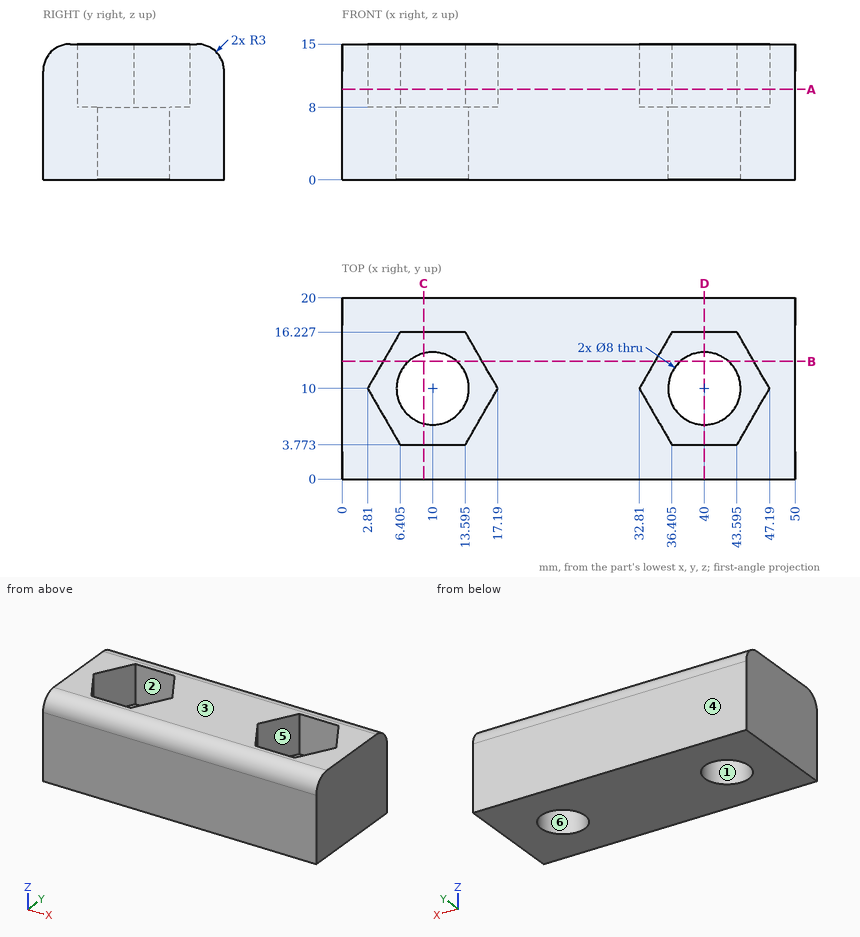
Can you work these out from the drawing? Everything is in mm from the part's minimum corner. A direction names the side the tool comes from. Coordinates: 2 decimals unless noted, no trailing zeros. Loops run counter-clockwise (first coordinate to the right, second up) from the corner with the lowest first, then second, coordinate; pieces in that order, holes last. Notation, with made-up numbers: M -17.75,69 L -10.75,69 A7 cw -10.75,80 Z; hole C 9.5,42.25 d9. An arc over 180 degrees is marked long. Put each result on its own line as item: value. Start each with the question number.
(1) Thinking about a two-plate mould opening in Y: for the marked faces 3, 4, 5 and 6, which applies, pulls with the +Y half, pulls with the -Y half, needs draft (parallel to the pull), parting line crosses it, or undercut?
(2) I need wall thicknesses on line 1 (X direction, y = 10, z = 10.5); line 2 (X direction, y = 10, z = 3); line 3 (Y direction, x = 42, z = 11.25). Which ranges of each line are inside material? Lowest first, please. Write a range as from..to.
(3) Will this pin go through, and if not, where does the flat tip stop? P1, Ø6, axis at x = 9, y = 9, coming from the +Z side.
(4) Suppose I cut it at B-B on y = 13. Please give me the cut outline in (x, z).
(5) For the marked faces 1 and 2, which set-ups out of +Z, -Z, +X, -X, +Y, -Y let a thin tool reach every point of the face, with its end or its side?
(6) Suppose I cut it at D-D on x = 40. Please give me the cut outline in (y, z), then the cut area to 3 significant figures.
(7) Suppose I cut it at C-C on x = 9. Please give me the cut outline in (y, z).
(8) Suppose I cut it at A-A on z = 10. Please give me the cut outline in (x, y) (1 decimal).
Solutions:
1. face 3: needs draft
1. face 4: pulls with the +Y half
1. face 5: undercut
1. face 6: undercut
2. line 1: x = 0..2.81, 17.19..32.81, 47.19..50
2. line 2: x = 0..6, 14..36, 44..50
2. line 3: y = 0..3.77, 16.23..20
3. P1: stops at z = 8
4. outline: M 0,0 L 7.35,0 L 7.35,8 L 4.54,8 L 4.54,15 L 0,15 Z; M 12.65,0 L 37.35,0 L 37.35,8 L 34.54,8 L 34.54,15 L 15.46,15 L 15.46,8 L 12.65,8 Z; M 42.65,0 L 50,0 L 50,15 L 45.46,15 L 45.46,8 L 42.65,8 Z
5. face 1: +Z, -Z
5. face 2: +Z
6. outline: M 0,0 L 6,0 L 6,8 L 3.77,8 L 3.77,15 L 3,15 A3 ccw 0,12 Z; M 14,0 L 20,0 L 20,12 A3 ccw 17,15 L 16.23,15 L 16.23,8 L 14,8 Z
6. area: 145 mm2
7. outline: M 0,0 L 6.13,0 L 6.13,8 L 3.77,8 L 3.77,15 L 3,15 A3 ccw 0,12 Z; M 13.87,0 L 20,0 L 20,12 A3 ccw 17,15 L 16.23,15 L 16.23,8 L 13.87,8 Z
8. outline: M 0,0 L 50,0 L 50,20 L 0,20 Z; hole M 2.8,10 L 6.4,3.8 L 13.6,3.8 L 17.2,10 L 13.6,16.2 L 6.4,16.2 Z; hole M 32.8,10 L 36.4,3.8 L 43.6,3.8 L 47.2,10 L 43.6,16.2 L 36.4,16.2 Z
